Work out the finished part from the listing and answer in its coordinate system (mm). Face numbers are marked on the shaded views. A direction names the side the tool comes from. Round coordinates to 2 decimals unless told otherwise and drop trailing zeros. Write each loop counter-clockwise with the first axis right and the second up, starting at its lowest first coordinate (ties: lowest second). Pieces come first, ordered by that corner, then holes.
1. Find section A-A (y = -8). Write down the section's boundary in (x, z), and give its area (3 significant figures).
2. Straight lines are drawn through the part: probe 1 along X at (y, z) = (0, 26); probe 2 along Y at (x, z) = (90, 32); probe 3 along Y at (x, z) = (90, 28.4). For each, find the intervals that lie inside material, in ascending order.
3. Find section B-B (x = 24). Write down the section's boundary in (y, z), and give its area (3 significant figures).
4. Flat-ended cylindrical pins translate along their axes: pin 1 Ø10 at (y, z) = (-9, 67.5) entering from -X; pin 2 Ø2 at (x, y) = (52, -44) entering from +Z; pin 3 Ø8 at (x, y) = (154.5, 18) entering from -Z; pin 4 Ø4 at (x, y) = (90, 0) entering from +Z. Find the tip coordinate at first contact, or state that the pin passes through.
5. Find section C-C (z = 131.5). Write down the section's boundary in (x, y), and give its area (3 significant figures).
6. Determine the mould class of the marked faces 4, 5 and 6 for opening direction Y: pulls with the +Y half, pulls with the -Y half, needs draft (parallel to the pull), parting line crosses it, or undercut.
7. A tool of negligible diameter and unlimited length cuts with its end or side. For the marked faces 1, 2 and 3, from which of +Z, -Z, +X, -X, +Y, -Y can it reach the whole face along a straight path? Write none if from no direction.
8. Find section D-D (y = 15.5). Write down the section's boundary in (x, z), and give its area (3 significant figures).
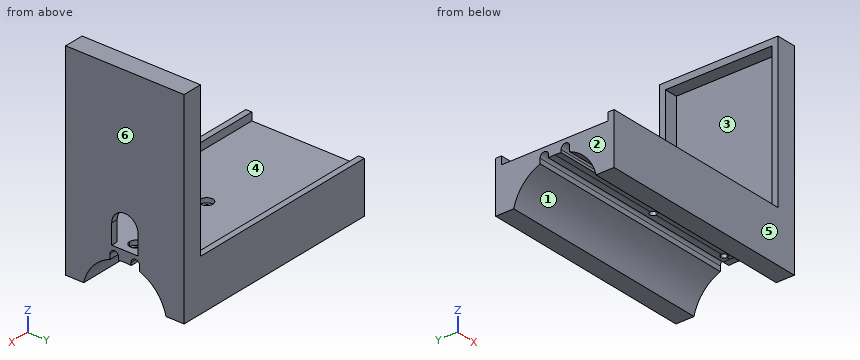
```python
from build123d import *

# Parameters (mm, degrees)
F1_DEPTH  = 160
F3_DEPTH  = 5
F4_W      = 4.5
F4_H      = 110.5
F5_DEPTH  = 10
F6_W      = 15
F6_H      = 90
F7_DEPTH  = 5
F8_R      = 2.5
F9_DEPTH  = 33.001
F8_R_2    = 4.7
F10_DEPTH = 3.5
F11_W     = 10
F11_H     = 15
F12_DEPTH = 5.0010001


with BuildPart() as f1:
    # F0 (on Right) → F1 (new body)
    with BuildSketch(Plane.YZ):
        with BuildLine():
            ThreePointArc((-4.75, 24.6467332166), (-2.3815922354, 24.9122273292), (0, 25.0008889767))
            Line((0, 25.0008889767), (0, 33))
            Line((0, 33), (-40.5, 33))
            Line((-40.5, 33), (-40.5, 39))
            Line((-40.5, 39), (-45, 39))
            Line((-45, 39), (-45, 0))
            Line((-45, 0), (-31.25, 0))
            ThreePointArc((-31.25, 0), (-24.152761856, 14.0086402639), (-11.25, 22.960261782))
            Line((-11.25, 22.960261782), (-11.25, 26.75))
            ThreePointArc((-11.25, 26.75), (-8, 30), (-4.75, 26.75))
            Line((-4.75, 26.75), (-4.75, 24.6467332166))
        make_face()
        with BuildLine():
            Line((0, 33), (0, 25.0008889767))
            ThreePointArc((0, 25.0008889767), (2.3815922354, 24.9122273292), (4.75, 24.6467332166))
            Line((4.75, 24.6467332166), (4.75, 26.75))
            ThreePointArc((4.75, 26.75), (8, 30), (11.25, 26.75))
            Line((11.25, 26.75), (11.25, 22.960261782))
            ThreePointArc((11.25, 22.960261782), (24.152761856, 14.0086402639), (31.25, 0))
            Line((31.25, 0), (45, 0))
            Line((45, 0), (45, 39))
            Line((45, 39), (40.5, 39))
            Line((40.5, 39), (40.5, 33))
            Line((40.5, 33), (0, 33))
        make_face()
    extrude(amount=F1_DEPTH)

    # F2 (on face) → F3 (join)
    with BuildSketch(Plane.YZ.offset(160)):
        with BuildLine():
            ThreePointArc((11.25, 22.960261782), (24.152761856, 14.0086402639), (31.25, 0))
            Line((31.25, 0), (45, 0))
            Line((45, 0), (45, 39))
            Line((45, 39), (40.5, 39))
            Line((40.5, 39), (40.5, 33))
            Line((40.5, 33), (-40.5, 33))
            Line((-40.5, 33), (-40.5, 39))
            Line((-40.5, 39), (-45, 39))
            Line((-45, 39), (-45, 0))
            Line((-45, 0), (-31.25, 0))
            ThreePointArc((-31.25, 0), (-24.152761856, 14.0086402639), (-11.25, 22.960261782))
            Line((-11.25, 22.960261782), (-11.25, 26.75))
            ThreePointArc((-11.25, 26.75), (-8, 30), (-4.75, 26.75))
            Line((-4.75, 26.75), (-4.75, 24.6467332166))
            ThreePointArc((-4.75, 24.6467332166), (0, 25.0008889767), (4.75, 24.6467332166))
            Line((4.75, 24.6467332166), (4.75, 26.75))
            ThreePointArc((4.75, 26.75), (8, 30), (11.25, 26.75))
            Line((11.25, 26.75), (11.25, 22.960261782))
        make_face()
        Polygon((40.5, 39), (45, 39), (45, 149.5), (-45, 149.5), (-45, 39), (-40.5, 39), (-40.5, 33), (40.5, 33), align=None)
    extrude(amount=F3_DEPTH)

    # F4 (on face) → F5 (join)
    with BuildSketch(Plane(origin=(160, 0, 0), x_dir=(0, -1, 0), z_dir=(-1, 0, 0))):
        with Locations((-42.75, 94.25)):
            Rectangle(F4_W, F4_H)
        with Locations((42.75, 94.25)):
            Rectangle(F4_W, F4_H)
    extrude(amount=F5_DEPTH)

    # F6 (on face) → F7 (join)
    with BuildSketch(Plane.XY.offset(149.5)):
        with Locations((157.5, 0)):
            Rectangle(F6_W, F6_H)
    extrude(amount=F7_DEPTH)

    # F8 (on face) → F9 (cut, through all)
    with BuildSketch(Plane.XY.offset(33)):
        with BuildLine():
            Line((155, 2.5), (155, -2.5))
            ThreePointArc((155, -2.5), (156.767766953, -1.767766953), (157.5, 0))
            ThreePointArc((157.5, 0), (156.767766953, 1.767766953), (155, 2.5))
        make_face()
        with BuildLine():
            ThreePointArc((155, 2.5), (152.5, 0), (155, -2.5))
            Line((155, -2.5), (155, 2.5))
        make_face()
        with Locations((90, 0)):
            Circle(F8_R)
    extrude(amount=-F9_DEPTH, mode=Mode.SUBTRACT)

    # F8 (on face) → F10 (cut)
    with BuildSketch(Plane.XY.offset(33)):
        with BuildLine():
            ThreePointArc((155, 4.7), (150.3, 0), (155, -4.7))
            Line((155, -4.7), (155, -2.5))
            ThreePointArc((155, -2.5), (152.5, 0), (155, 2.5))
            Line((155, 2.5), (155, 4.7))
        make_face()
        with BuildLine():
            Line((155, -2.5), (155, -4.7))
            ThreePointArc((155, -4.7), (158.3234018716, -3.3234018716), (159.7, 0))
            ThreePointArc((159.7, 0), (158.3234018716, 3.3234018716), (155, 4.7))
            Line((155, 4.7), (155, 2.5))
            ThreePointArc((155, 2.5), (156.767766953, 1.767766953), (157.5, 0))
            ThreePointArc((157.5, 0), (156.767766953, -1.767766953), (155, -2.5))
        make_face()
        with Locations((90, 0)):
            Circle(F8_R_2)
        with Locations((90, 0)):
            Circle(F8_R, mode=Mode.SUBTRACT)
    extrude(amount=-F10_DEPTH, mode=Mode.SUBTRACT)

    # F11 (on face) → F12 (cut, through all)
    with BuildSketch(Plane(origin=(160, 0, 0), x_dir=(0, -1, 0), z_dir=(-1, 0, 0))):
        with Locations((5, 40.5)):
            Rectangle(F11_W, F11_H)
        with Locations((-5, 40.5)):
            Rectangle(F11_W, F11_H)
        with BuildLine():
            Line((0, 48), (10, 48))
            ThreePointArc((10, 48), (7.071067816, 55.0710678077), (1.18e-08, 58))
            Line((0, 58), (0, 48))
        make_face()
        with BuildLine():
            Line((-10, 48), (0, 48))
            Line((0, 48), (0, 58))
            ThreePointArc((1.18e-08, 58), (-7.0710678077, 55.071067816), (-10, 48))
        make_face()
    extrude(amount=-F12_DEPTH, mode=Mode.SUBTRACT)


solid = f1.part
```
Worked answers:
1. outline: (0, 30) - (165, 30) - (165, 33) - (0, 33) - close; (150, 149.5) - (160, 149.5) - (160, 54) - (165, 54) - (165, 154.5) - (150, 154.5) - close
1. area: 1,050 mm2
2. probe 1: x = 0 to 87.5, 92.5 to 152.5, 157.5 to 165
2. probe 2: y = -45 to -4.7, 4.7 to 45
2. probe 3: y = -45 to -10.8, -5.2 to -2.5, 2.5 to 5.2, 10.8 to 45
3. outline: (-45, 0) - (-31.25, 0) arc R32.03 cw to (-11.25, 22.96) - (-11.25, 26.75) arc R3.25 cw to (-4.75, 26.75) - (-4.75, 24.65) arc R32.03 cw to (4.75, 24.65) - (4.75, 26.75) arc R3.25 cw to (11.25, 26.75) - (11.25, 22.96) arc R32.03 cw to (31.25, 0) - (45, 0) - (45, 39) - (40.5, 39) - (40.5, 33) - (-40.5, 33) - (-40.5, 39) - (-45, 39) - close
3. area: 1,790 mm2
4. pin 1: stops at x = 160
4. pin 2: stops at z = 39
4. pin 3: stops at z = 16.25
4. pin 4: passes through
5. outline: (150, -45) - (165, -45) - (165, 45) - (150, 45) - (150, 40.5) - (160, 40.5) - (160, -40.5) - (150, -40.5) - close
5. area: 540 mm2
6. face 4: undercut
6. face 5: pulls with the -Y half
6. face 6: needs draft
7. face 1: -Z, +X, -X
7. face 2: +Z, -Z, -X, +Y, -Y
7. face 3: -X
8. outline: (0, 21) - (165, 21) - (165, 154.5) - (150, 154.5) - (150, 149.5) - (160, 149.5) - (160, 33) - (0, 33) - close
8. area: 2,640 mm2
